from build123d import *

# Parameters (mm, degrees)
SKETCH1_R           = 25
BOSS_EXTRUDE1_DEPTH = 356.5
SKETCH2_R           = 27.5
BOSS_EXTRUDE2_DEPTH = 30
SKETCH3_R           = 27.5
BOSS_EXTRUDE3_DEPTH = 30
SKETCH4_R           = 6.7
CUT_EXTRUDE1_DEPTH  = 20
SKETCH5_R           = 6.7
CUT_EXTRUDE2_DEPTH  = 20
SKETCH6_R           = 6.7
CUT_EXTRUDE3_DEPTH  = 20
FILLET1_R           = 1


with BuildPart() as part:
    # Sketch1 → Boss-Extrude1 (new body)
    with BuildSketch(Plane(origin=(0, 0, 0), x_dir=(0, 1, 0), z_dir=(0, 0, 1))):
        Circle(SKETCH1_R)
    extrude(amount=BOSS_EXTRUDE1_DEPTH)

    # Sketch2 → Boss-Extrude2 (add)
    with BuildSketch(Plane.XY.offset(356.5)):
        Circle(SKETCH2_R)
    extrude(amount=-BOSS_EXTRUDE2_DEPTH)

    # Sketch3 → Boss-Extrude3 (add)
    with BuildSketch(Plane(origin=(0, 0, 0), x_dir=(-1, 0, 0), z_dir=(0, 0, -1))):
        Circle(SKETCH3_R)
    extrude(amount=-BOSS_EXTRUDE3_DEPTH)

    # Sketch4 → Cut-Extrude1 (cut)
    with BuildSketch(Plane(origin=(0, 0, 0), x_dir=(1, 0, 0), z_dir=(0, 0, -1))):
        Circle(SKETCH4_R)
    extrude(amount=-CUT_EXTRUDE1_DEPTH, mode=Mode.SUBTRACT)

    # Sketch5 → Cut-Extrude2 (cut)
    with BuildSketch(Plane.XY.offset(356.5)):
        Circle(SKETCH5_R)
    extrude(amount=-CUT_EXTRUDE2_DEPTH, mode=Mode.SUBTRACT)

    # Sketch6 → Cut-Extrude3 (cut)
    with BuildSketch(Plane(origin=(0, 25, 0), x_dir=(-1, 0, 0), z_dir=(0, 1, 0))):
        with Locations((0, 70)):
            Circle(SKETCH6_R)
    extrude(amount=-CUT_EXTRUDE3_DEPTH, mode=Mode.SUBTRACT)

    # Fillet1
    fillet1_edges = [part.edges().sort_by_distance(p)[0] for p in [
        (27.5, 0, 30),
        (27.5, 0, 0),
        (-27.5, 0, 326.5),
        (-27.5, 0, 356.5),
    ]]
    fillet(fillet1_edges, radius=FILLET1_R)


solid = part.part
Read the model definition and answer for the solid it produces. Units are mm, in the model's axes. A direction names the side the tool comes from. Round coordinates to 2 decimals unless told otherwise and drop trailing zeros. Order: outer loops, then holes, each group sorted by start corner. A loop starts at its lowest first (then second) coordinate and runs counter-clockwise, first axis right, second up.
1) For faces 4 (the face through (-6.694, -0.295, 9.86)), 5 (the face through (-6.694, 0.295, 346.64)), 6 (the face through (0, 5, 70)), 7 (the face through (20, 16, 326.5)), determine the directions among +Z, -Z, +X, -X, +Y, -Y from which every point of the face is accessible in a straight line to the end or side of a thin tool.
2) The part is cut by section A-A on y = 0. Write down the section's boundary in (x, z), plus the area to 3 significant figures.
3) The mould has two halves that part along X. Classify faces 1 (the face through (5.961, -26.846, 14.804)), 2 (the face through (-6, -6, 0)), 3 (the face through (1.45, 15.14, 63.46)): released by +X, released by -X, zero draft, split by the parting line, or undercut.
4) The part is cut by section C-C on z = 239. Write down the section's boundary in (x, y), plus the area to 3 significant figures.
5) Straight lines are drawn through the part: L1, parallel to Y at x = 0, z = 9; L2, parallel to Z at x = 2.5, y = -3; L3, parallel to X at y = 12.25, z = 70. For each, find the intervals that lie inside material, in ascending order.
6) Flat-ended cylindrical pins translate along their axes: pin 1 (4 mm diameter, centred on x = -2, y = 1, fed in from -Z); pin 2 (10 mm diameter, centred on x = -12, z = 269, fed in from +Y); pin 3 (6 mm diameter, centred on x = 12.5, z = 210, fed in from +Y). Find the tip coordinate at first contact, or state that the pin passes through.
7) The part is cut by section D-D on z = 70. Write down the section's boundary in (x, y).
Resolved:
1. face 4: -Z
1. face 5: +Z
1. face 6: +Y
1. face 7: none
2. outline: (-27.5, 1) arc R1 ccw to (-26.5, 0) - (-6.7, 0) - (-6.7, 20) - (6.7, 20) - (6.7, 0) - (26.5, 0) arc R1 ccw to (27.5, 1) - (27.5, 29) arc R1 ccw to (26.5, 30) - (25, 30) - (25, 326.5) - (26.5, 326.5) arc R1 ccw to (27.5, 327.5) - (27.5, 355.5) arc R1 ccw to (26.5, 356.5) - (6.7, 356.5) - (6.7, 336.5) - (-6.7, 336.5) - (-6.7, 356.5) - (-26.5, 356.5) arc R1 ccw to (-27.5, 355.5) - (-27.5, 327.5) arc R1 ccw to (-26.5, 326.5) - (-25, 326.5) - (-25, 30) - (-26.5, 30) arc R1 ccw to (-27.5, 29) - close
2. area: 17,600 mm2
3. face 1: split by the parting line
3. face 2: zero draft
3. face 3: undercut
4. outline: circle Ø50 at (0, 0)
4. area: 1,960 mm2
5. L1: y = -27.5 to -6.7, 6.7 to 27.5
5. L2: z = 20 to 336.5
5. L3: x = -21.79 to -6.7, 6.7 to 21.79
6. pin 1: stops at z = 20
6. pin 2: stops at y = 24
6. pin 3: stops at y = 23.12
7. outline: (-6.7, 5) - (-6.7, 24.09) arc R25 ccw (long way) to (6.7, 24.09) - (6.7, 5) - close
